Geometry: see drawing. Coordinates: mm, zero at the bounding-box minimum. A direction names the side the tool comes from. Round coordinates to 2 decimals unless told otherwise and drop trailing zeros. Loops run counter-clockwise (first coordinate to the right, second up) from the corner with the lowest first, then second, coordinate; pieces in that order, holes last. Notation, with made-up numbers: (-36, 53) - (-20, 53) arc R17 ccw to (-20, 61) - close; hole circle Ø9 at (19.5, 39.25). An arc over 180 degrees is marked (long way). Return JSON: item names as keys, results as strings. Group by question number.
1. Set-up query: the marked faces 1 and 2. Return all of +Z, -Z, +X, -X, +Y, -Y with unobstructed straight access to the full face (end or side cutting, diameter ignored); none if empty.
2. Material intervals for probe 1 along Y at (x, z) = (4.5, 0.2); probe 2 along X at (y, z) = (4, 0.45); probe 3 along Y at (x, z) = (3, 3), sorted ascending.
3. Section C-C on z = 1.5. Return loops of the section in (x, y) (1 decimal).
4. Section D-D on y = 7.5. Return loops of the section in (x, z) (1 decimal), and give its area (3 significant figures).
5. First-contact query: pin 1 Ø1.6 at (x, y) = (5.5, 3) entering from +Z; pin 2 Ø0.8 at (y, z) = (3.5, 2) entering from -X (1 decimal); pin 3 Ø1.5 at (y, z) = (3.5, 1.5) entering from +X. Flat tips, straight axial feed; report the tip coordinate or a pass-through.
6. Draft query along Y for the marked faces 3, 4, 5 and 6. Return one class per face: +Y half, -Y half, draft (parallel to the pull), parting line (faces both ways), or undercut.
7. Section A-A on y = 4. Return loops of the section in (x, z) (1 decimal), and give its area (3 significant figures).
8. Section B-B on x = 5.25. Return loops of the section in (y, z) (1 decimal).
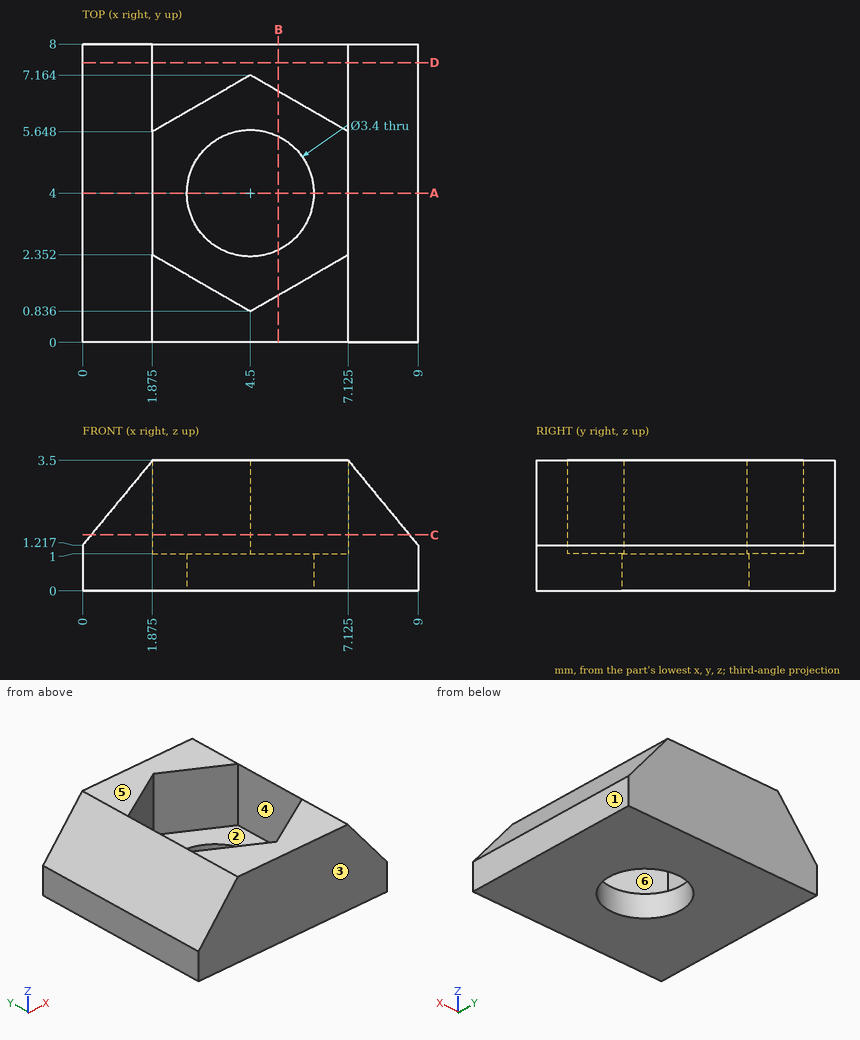
Taken from the geometry:
{
 "1": {"face 1": "+Z, -Z, +X, +Y, -Y", "face 2": "+Z"},
 "2": {"probe 1": "0 to 2.3, 5.7 to 8", "probe 2": "0 to 2.8, 6.2 to 9", "probe 3": "0 to 1.7, 6.3 to 8"},
 "3": {"outline": "(0.2, 0) - (8.8, 0) - (8.8, 8) - (0.2, 8) - close; hole (1.9, 2.4) - (4.5, 0.8) - (7.1, 2.4) - (7.1, 5.6) - (4.5, 7.2) - (1.9, 5.6) - close"},
 "4": {"outline": "(0, 0) - (9, 0) - (9, 1.2) - (7.1, 3.5) - (1.9, 3.5) - (0, 1.2) - close", "area": "27.2 mm2"},
 "5": {"pin 1": "z = 1", "pin 2": "x = 0.3", "pin 3": "x = 9"},
 "6": {"face 3": "-Y half", "face 4": "undercut", "face 5": "draft", "face 6": "undercut"},
 "7": {"outline": "(0, 0) - (2.8, 0) - (2.8, 1) - (1.9, 1) - (1.9, 3.5) - (0, 1.2) - close; (6.2, 0) - (9, 0) - (9, 1.2) - (7.1, 3.5) - (7.1, 1) - (6.2, 1) - close", "area": "10.7 mm2"},
 "8": {"outline": "(0, 0) - (2.5, 0) - (2.5, 1) - (1.3, 1) - (1.3, 3.5) - (0, 3.5) - close; (5.5, 0) - (8, 0) - (8, 3.5) - (6.7, 3.5) - (6.7, 1) - (5.5, 1) - close"}
}
